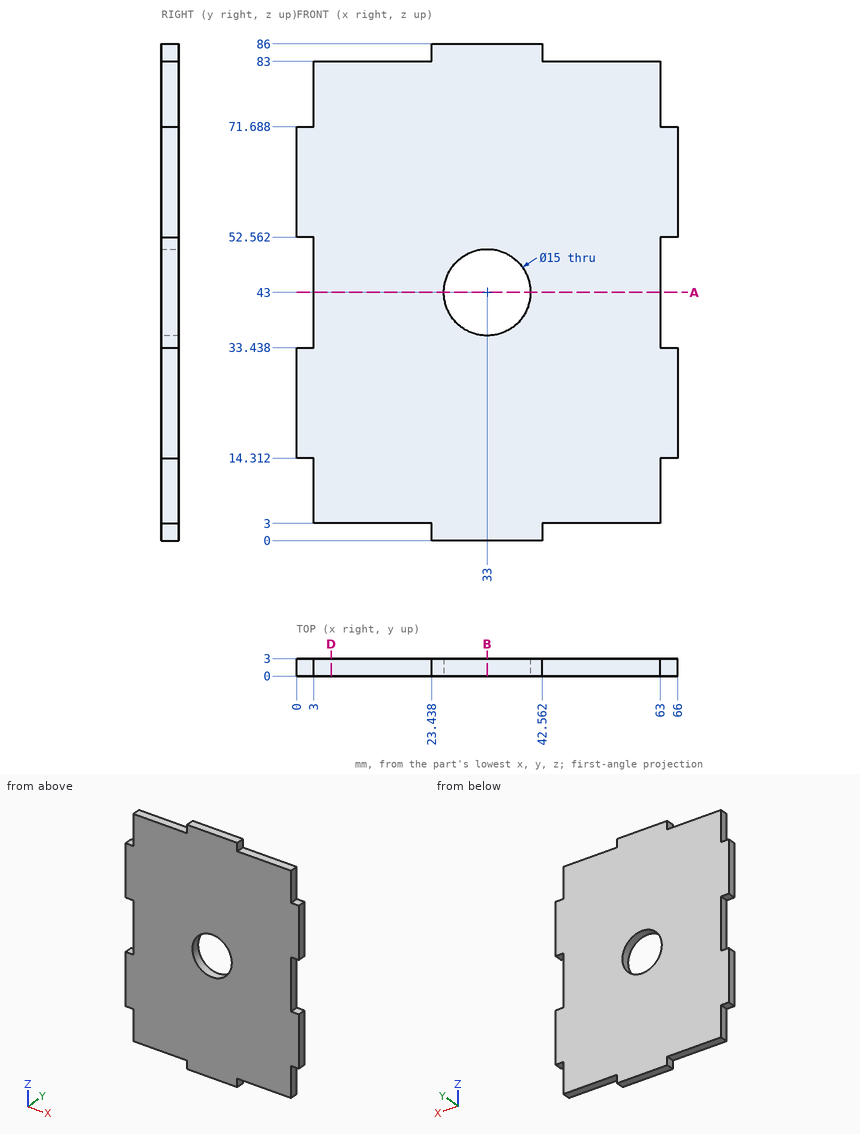
Verification items for this drawing (mm, ordinates from the low corner). Coordinates: 2 decimals unless noted, no trailing zeros. Order: outer loops, then holes, each group sorted by start corner. A loop starts at its lowest first (then second) coordinate and runs counter-clockwise, first axis right, second up. Notation, with made-up numbers: M 62.5,81.5 L 112.5,81.5 A16 cw 112.5,88.5 Z; hole C 36.25,31 d1. An arc over 180 degrees is marked long. Write each question's results on one line, items separated by ' | '.
1) Section check B-B on x = 33. Record the cut outline in (y, z).
Solved:
outline: M 0,0 L 3,0 L 3,35.5 L 0,35.5 Z; M 0,50.5 L 3,50.5 L 3,86 L 0,86 Z
2) Gauge pin test, flat ends, axial feed: pin 1 Ø1.5 at (x, y) = (12, 2) entering from +Z; pin 2 Ø0.9 at (y, z) = (1, 85) entering from -X; pin 3 Ø0.9 at (x, y) = (1.5, 1.5) entering from +Z. Record the tip position at first contact, or that the pin passes through.
Solved:
pin 1: stops at z = 83 | pin 2: stops at x = 23.44 | pin 3: stops at z = 71.69
3) Section check A-A on z = 43. Record the cut outline in (x, y), plus the area to 3 significant figures.
Solved:
outline: M 3,0 L 25.5,0 L 25.5,3 L 3,3 Z; M 40.5,0 L 63,0 L 63,3 L 40.5,3 Z | area: 135 mm²
4) Section check D-D on x = 6. Record the cut outline in (y, z).
Solved:
outline: M 0,3 L 3,3 L 3,83 L 0,83 Z
5) Scan lines: line 1 along X through (y, z) = (2.1, 43); line 2 along Z through (x, y) = (18, 1.5); line 3 along X through (y, z) = (2.1, 80). Record each from-to range of solid material in increasing order. Write a range as [from, to].
Solved:
line 1: x = [3, 25.5], [40.5, 63] | line 2: z = [3, 83] | line 3: x = [3, 63]
